Read the model definition and answer for the solid it produces. Units are mm, in the model's axes. A direction names the side the tool comes from. Coordinates: 2 decimals unless noted, no trailing zeros. Order: outer loops, then holes, each group sorted by start corner. A loop starts at its lowest first (then second) coordinate and runs counter-clockwise, first axis right, second up. Notation, with made-up numbers: (84.25, -35) - (123.25, -35) arc R30 cw to (123.25, -13) - close; hole circle Ø11 at (-5.5, 62). An arc over 180 degrees is marked (long way). Use one line per item in the form item = value.
```python
from build123d import *

# Parameters (mm, degrees)
EXTRUDE_THIN1_DEPTH = 365.125
FILLET1_R           = 1.27


with BuildPart() as part:
    # Sketch1 → Extrude-Thin1 (new body)
    with BuildSketch(Plane.XY):
        with BuildLine():
            Line((-0.396875, 6.35), (0, 0))
            Line((0, 0), (-6.35, 0))
            Line((-6.35, 0), (-6.35, 3.175))
            ThreePointArc((-6.35, 3.175), (-9.717596045, 4.569903955), (-11.1125, 7.9375))
            Line((-11.1125, 7.9375), (-11.1125, 11.1125))
            Line((-11.1125, 11.1125), (-12.7, 11.1125))
            Line((-12.7, 11.1125), (-12.7, 26.9875))
            ThreePointArc((-12.7, 26.9875), (-14.094903955, 30.355096045), (-17.4625, 31.75))
            Line((-17.4625, 31.75), (-17.4625, 36.5125))
            Line((-17.4625, 36.5125), (-3.175, 36.5125))
            Line((-3.175, 36.5125), (-3.175, 35.2425))
            Line((-3.175, 35.2425), (-16.1925, 35.2425))
            Line((-16.1925, 35.2425), (-16.1925, 32.88480076))
            ThreePointArc((-16.1925, 32.88480076), (-12.769295804, 30.777604303), (-11.43, 26.9875))
            Line((-11.43, 26.9875), (-11.43, 12.3825))
            Line((-11.43, 12.3825), (-9.8425, 12.3825))
            Line((-9.8425, 12.3825), (-9.8425, 7.9375))
            ThreePointArc((-9.8425, 7.9375), (-8.320035691, 5.053663038), (-5.08, 4.684093132))
            Line((-5.08, 4.684093132), (-5.08, 1.27))
            Line((-5.08, 1.27), (-1.351853051, 1.27))
            Line((-1.351853051, 1.27), (-1.664401775, 6.270779577))
            Line((-1.664401775, 6.270779577), (-0.396875, 6.35))
        make_face()
    extrude(amount=-EXTRUDE_THIN1_DEPTH)

    # Fillet1
    fillet1_edges = [part.edges().sort_by_distance(p)[0] for p in [
        (-9.8425, 12.3825, -182.5625),
        (-5.08, 4.684093132, -182.5625),
        (0, 0, -182.5625),
        (-6.35, 0, -182.5625),
        (-12.7, 11.1125, -182.5625),
        (-17.4625, 31.75, -182.5625),
        (-17.4625, 36.5125, -182.5625),
    ]]
    fillet(fillet1_edges, radius=FILLET1_R)


solid = part.part
```
(1) Section B-B, the plane y = 18 is taken. Write down the section's boundary in (x, z) (3 decimals), then the cut area to 3 significant figures.
Answer list:
outline = (-12.7, -365.125) - (-11.43, -365.125) - (-11.43, 0) - (-12.7, 0) - close
area = 464 mm2
(2) The mould has two halves that part along Y. Classify faces 1 (the flat face through (-11.43, 20, -180)), 2 (the flat face through (-10, 36.512, -180)), 3 (the flat face through (-12, 18, -365.125)): +Y half, -Y half, draft (parallel to the pull), parting line (faces both ways), or undercut.
Answer list:
face_1 = undercut
face_2 = +Y half
face_3 = draft
(3) Which of the six approach directions +Z, -Z, +X, -X, +Y, -Y give full straight-line access (tool end or side, diameter ignored) to faces 4 (the flat face through (-12.7, 20, -180)), 5 (the cylindrical face through (-12.806, 30.822, -180.007)), 6 (the flat face through (-12, 18, 0))?
Answer list:
face_4 = +Z, -Z, -X, -Y
face_5 = +Z, -Z, +X
face_6 = +Z, +X, -X, +Y, -Y
(4) Given pin 1 Ø16 at (y, z) = (19.5, -262.5) entering from -X; pin 2 Ø8 at (x, z) = (-10.5, -305.5) entering from -Y; pin 3 Ø0.7 at (y, z) = (34, -110.5) entering from +X, each flat-ended and moving along its own axis, determine where each tip first touches the part or whether it passes through.
Answer list:
pin_1 = -12.73
pin_2 = 3.18
pin_3 = -16.19
(5) Straight lines are drawn through the part: L1, parallel to Y at x = -7, z = -145.5; L2, parallel to X at y = 2, z = -244.5 (3 decimals); L3, parallel to Y at x = -15.5, z = -291. For each, find the intervals that lie inside material, in ascending order.
Answer list:
L1 = 3.22 to 4.51, 35.24 to 36.51
L2 = -6.35 to -5.08, -1.397 to -0.125
L3 = 31.33 to 32.69, 35.24 to 36.51
